```python
from build123d import *

# Parameters (mm, degrees)
SKETCH1_W                = 50
SKETCH1_H                = 40
BOSS_EXTRUDE1_DEPTH      = 20
SKETCH2_R                = 5
BOSS_EXTRUDE2_DEPTH      = 5
BOSS_EXTRUDE2_DEPTH_BACK = 55


with BuildPart() as part:
    # Sketch1 → Boss-Extrude1 (new body)
    with BuildSketch(Plane.XY):
        Rectangle(SKETCH1_W, SKETCH1_H)
    extrude(amount=BOSS_EXTRUDE1_DEPTH)

    # Sketch2 → Boss-Extrude2 (add, two sides)
    with BuildSketch(Plane.ZY.offset(25)) as boss_extrude2_sk:
        with Locations((10, 10.407747154)):
            Circle(SKETCH2_R)
    extrude(amount=BOSS_EXTRUDE2_DEPTH)
    extrude(boss_extrude2_sk.sketch, amount=-BOSS_EXTRUDE2_DEPTH_BACK)


solid = part.part
```
Could you check a few things on this model? Use its own coordinates, in mm. A direction names the side the tool comes from. Coordinates: 2 decimals unless noted, no trailing zeros. Write each loop counter-clockwise with the first axis right and the second up, starting at its lowest first coordinate (ties: lowest second). Pieces come first, ordered by that corner, then holes. Notation, with made-up numbers: (70.5, -3.75) -> (89.5, -3.75) arc R5 cw to (89.5, 5.25) -> close; hole circle Ø4 at (15, -34.5). An arc over 180 degrees is marked (long way). Return JSON: item names as keys, results as strings.
(1) Imagine slicing it at D-D, the plane z = 4. Please give me the cut outline in (x, y).
Numbers:
{"outline": "(-25, -20) -> (25, -20) -> (25, 20) -> (-25, 20) -> close"}
(2) Imagine slicing it at C-C, the plane z = 7.25. Please give me the cut outline in (x, y).
Numbers:
{"outline": "(-30, 6.23) -> (-25, 6.23) -> (-25, -20) -> (25, -20) -> (25, 6.23) -> (30, 6.23) -> (30, 14.58) -> (25, 14.58) -> (25, 20) -> (-25, 20) -> (-25, 14.58) -> (-30, 14.58) -> close"}
(3) I need wall thicknesses on L1, parallel to X at y = 4, z = 16; L2, parallel to Z at x = -25.5, y = 11.5. Which ranges of each line are inside material? Lowest first, please.
Numbers:
{"L1": "x = -25 to 25", "L2": "z = 5.12 to 14.88"}
(4) Imagine slicing it at A-A, the plane z = 10. Please give me the cut outline in (x, y), then the cut area to 3 significant figures.
Numbers:
{"outline": "(-30, 5.41) -> (-25, 5.41) -> (-25, -20) -> (25, -20) -> (25, 5.41) -> (30, 5.41) -> (30, 15.41) -> (25, 15.41) -> (25, 20) -> (-25, 20) -> (-25, 15.41) -> (-30, 15.41) -> close", "area": "2,100 mm2"}
(5) I'm going to push flat-ended pins straight in: pin 1 (3 mm diameter, centred on y = 5, z = 6, fed in from -X); pin 2 (1.5 mm diameter, centred on y = 1.5, z = 9.5, fed in from +X). Where does each tip first touch, or does it pass through?
Numbers:
{"pin 1": "stops at x = -25", "pin 2": "stops at x = 25"}
(6) Imagine slicing it at B-B, the plane y = -12. Please give me the cut outline in (x, z).
Numbers:
{"outline": "(-25, 0) -> (25, 0) -> (25, 20) -> (-25, 20) -> close"}
(7) Which directions (+Z, -Z, +X, -X, +Y, -Y) give clear straight access to the entire face, cutting with the end or side of a thin tool? Please do faces 1 (the cylindrical face through (-27.46, 11.91, 14.77)), 2 (the cylindrical face through (27.47, 11.91, 14.77)), 3 (the flat face through (0, 0, 20)).
Numbers:
{"face 1": "-X", "face 2": "+X", "face 3": "+Z, +X, -X, +Y, -Y"}
